Source: CAD feature listing. Evaluate the final solid. Frame: model axes, mm. A direction names the side the tool comes from. Give positions to 0.01 mm unless a question says otherwise; leave off trailing zeros. Order: outer loops, then holes, each group sorted by start corner. A loop starts at its lowest first (then second) coordinate and runs counter-clockwise, first axis right, second up. Notation, with made-up numbers: (36.5, 74) -> (71.5, 74) arc R17 cw to (71.5, 78) -> close; hole circle Ø2 at (2.5, 89). An arc over 180 degrees is marked (long way). Answer in a Markdown table with one row per item.
```python
from build123d import *

# Parameters (mm, degrees)
F0_W     = 95
F0_H     = 31
F0_W_2   = 69
F0_H_2   = 24
F1_DEPTH = 3
F2_DEPTH = 5.6
F3_R     = 1.5
F4_R     = 2.5
F5_DEPTH = 25
F6_SIZE  = 1.5


with BuildPart() as f1:
    # F0 (on Top) → F1 (new body)
    with BuildSketch(Plane.XY):
        with Locations((7.447391, -15.3567)):
            Rectangle(F0_W, F0_H)
        with Locations((7.447391, -16.8567)):
            Rectangle(F0_W_2, F0_H_2, mode=Mode.SUBTRACT)
    extrude(amount=F1_DEPTH)

    # F0 (on Top) → F2 (join)
    with BuildSketch(Plane.XY):
        with Locations((7.447391, -16.8567)):
            Rectangle(F0_W_2, F0_H_2)
    extrude(amount=F2_DEPTH)

    # F3
    f3_edges = [f1.edges().sort_by_distance(p)[0] for p in [
        (-40.052609, -15.3567, 0),
        (7.447391, 0.1433, 0),
        (7.447391, -30.8567, 0),
        (54.947391, -15.3567, 0),
    ]]
    fillet(f3_edges, radius=F3_R)

    # F4 (on face) → F5 (cut)
    with BuildSketch(Plane.XY.offset(5.6)):
        with Locations((-32.552609, -10.3567)):
            Circle(F4_R)
        with Locations((-32.552609, -23.3567)):
            Circle(F4_R)
        with Locations((47.447391, -23.3567)):
            Circle(F4_R)
        with Locations((47.447391, -10.3567)):
            Circle(F4_R)
    extrude(amount=-F5_DEPTH, mode=Mode.SUBTRACT)

    # F6
    f6_edges = [f1.edges().sort_by_distance(p)[0] for p in [
        (-38.552609, -15.3567, 0),
        (7.447391, -1.3567, 0),
        (7.447391, -29.3567, 0),
        (53.447391, -15.3567, 0),
        (-35.052609, -23.3567, 0),
        (44.947391, -23.3567, 0),
        (-35.052609, -10.3567, 0),
        (44.947391, -10.3567, 0),
    ]]
    chamfer(f6_edges, length=F6_SIZE)


solid = f1.part
```
(1) First-contact query: pin 1 Ø0.8 at (x, z) = (23.5, 5) entering from +Y; pin 2 Ø6 at (x, y) = (-32.55, -23.36) entering from +Z. Flat tips, straight axial feed; report the tip coordinate or a pass-through.
A:
| item | result |
|---|---|
| pin 1 | stops at y = -4.86 |
| pin 2 | stops at z = 3 |
(2) Section query B-B (y = -17). Return the cut outline in (x, z).
A:
| item | result |
|---|---|
| outline | (-40.05, 1.5) arc R1.5 ccw to (-38.55, 0) -> (53.45, 0) arc R1.5 ccw to (54.95, 1.5) -> (54.95, 3) -> (41.95, 3) -> (41.95, 5.6) -> (-27.05, 5.6) -> (-27.05, 3) -> (-40.05, 3) -> close |
(3) Pull-direction query (X, two-part tool) for faces 1 (the flat face through (7, -4.857, 4)), 2 (the flat face through (41.947, -17, 4)), 3 (the cylindrical face through (49.832, -9.606, 2.26)); classes: +X half, -X half, draft (parallel to the pull), parting line (faces both ways), or undercut.
A:
| item | result |
|---|---|
| face 1 | draft |
| face 2 | +X half |
| face 3 | undercut |
(4) Section query A-A (x = -17). Return the cut outline in (y, z), plus the area to 3 significant figures.
A:
| item | result |
|---|---|
| outline | (-30.86, 1.5) arc R1.5 ccw to (-29.36, 0) -> (-1.36, 0) arc R1.5 ccw to (0.14, 1.5) -> (0.14, 3) -> (-4.86, 3) -> (-4.86, 5.6) -> (-28.86, 5.6) -> (-28.86, 3) -> (-30.86, 3) -> close |
| area | 154 mm^2 |
(5) Section query C-C (y = -25). Give the number of separate pieces and of enclosed holes in the cut face, plus the area to 3 significant figures.
A:
| item | result |
|---|---|
| separate pieces | 3 |
| enclosed holes | 0 |
| area | 435 mm^2 |
(6) Ray query, probe 1 along X at (y, z) = (-24, 0.55); probe 2 along X at (y, z) = (-24.5, 1.15); probe 3 along X at (y, z) = (-5.5, 3.55). Return the intervals inside material, ascending.
A:
| item | result |
|---|---|
| probe 1 | x = -39.71 to -35.94, -29.16 to 44.06, 50.84 to 54.61 |
| probe 2 | x = -40.01 to -35.16, -29.94 to 44.84, 50.06 to 54.91 |
| probe 3 | x = -27.05 to 41.95 |
(7) Access query for faces 4 (the cylindrical face through (-30.168, -9.606, 2.26)), 5 (the flat face through (7, -28.857, 4)), 6 (the flat face through (-27.053, -17, 4)). Directions: +Z, -Z, +X, -X, +Y, -Y. A direction counts if a zero-diameter tool reaches every point of the face in a straight line with its end or side. Return the directions, or none.
A:
| item | result |
|---|---|
| face 4 | +Z, -Z |
| face 5 | +Z, +X, -X, -Y |
| face 6 | +Z, -X, +Y, -Y |
